For this review, take the finished solid that the model builds, in its own axes (mm). A direction names the side the tool comes from. Coordinates: 2 decimals unless noted, no trailing zeros. Order: outer loops, then holes, each group sorted by start corner. A loop starts at its lowest first (then second) coordinate and runs counter-clockwise, first axis right, second up. Notation, with made-up numbers: M 31.25,-31 L 42.25,-31 A34 cw 42.25,5 Z; hole C -1.5,17 d7. An arc over 180 degrees is marked long. Use CSV: the item, a comma, the result in double quotes.
```python
from build123d import *

# Parameters (mm, degrees)
EXTRUDE_1_DEPTH          = 5
SKETCH_2_W               = 67
SKETCH_2_H               = 34
EXTRUDE_2_DEPTH          = 5
SKETCH_4_W               = 57
SKETCH_4_H               = 57
EXTRUDE_3_DEPTH          = 5
CUT_EXTRUDE_1_DEPTH      = 5
FILLET_1_R               = 10
FILLET_2_R               = 10
SKETCH_6_R               = 1.25
SKETCH_6_R_2             = 12.5
CUT_EXTRUDE_2_DEPTH      = 5
PATTERN_CIRCULAR_1_COUNT = 4
SKETCH_7_R               = 1.25
CUT_EXTRUDE_3_DEPTH      = 5
SKETCH_8_R               = 1.25
CUT_EXTRUDE_5_DEPTH      = 10
PATTERN_CIRCULAR_2_COUNT = 3
PATTERN_CIRCULAR_2_ANGLE = 180


with BuildPart() as part:
    # 草图1 → 凸台-拉伸1 (new body)
    with BuildSketch(Plane.XY):
        Polygon((23, 17), (28, 17), (28, -17), (23, -17), (-5, -17), (-5, 17), align=None)
    extrude(amount=EXTRUDE_1_DEPTH)

    # 草图2 → 凸台-拉伸2 (add)
    with BuildSketch(Plane(origin=(28, 0, 0), x_dir=(0, 0, -1), z_dir=(1, 0, 0))):
        with Locations((-38.5, 0)):
            Rectangle(SKETCH_2_W, SKETCH_2_H)
    extrude(amount=-EXTRUDE_2_DEPTH)

    # 草图4 → 凸台-拉伸3 (add)
    with BuildSketch(Plane.ZY.offset(-23)):
        with Locations((43.5, 0)):
            Rectangle(SKETCH_4_W, SKETCH_4_H)
    extrude(amount=-EXTRUDE_3_DEPTH)

    # 草图5 → 切除-拉伸1 (cut)
    with BuildSketch(Plane.ZY.offset(-23)):
        with BuildLine():
            Line((15, 28.5), (15, 17))
            Line((15, 17), (20.625341533, 17))
            ThreePointArc((20.625341533, 17), (30.698632886, 25.463208753), (43.5, 28.5))
            Line((43.5, 28.5), (15, 28.5))
        make_face()
        with BuildLine():
            ThreePointArc((43.500000073, -28.5), (30.698632918, -25.463208769), (20.625341533, -17))
            Line((20.625341533, -17), (15, -17))
            Line((15, -17), (15, -28.5))
            Line((15, -28.5), (43.500000073, -28.5))
        make_face()
        with BuildLine():
            ThreePointArc((72, 0), (63.65254329, -20.152543238), (43.500000073, -28.5))
            Line((43.500000073, -28.5), (72, -28.5))
            Line((72, -28.5), (72, 0))
        make_face()
        with BuildLine():
            Line((72, 28.5), (43.5, 28.5))
            ThreePointArc((43.5, 28.5), (63.652543264, 20.152543264), (72, 0))
            Line((72, 0), (72, 28.5))
        make_face()
    extrude(amount=-CUT_EXTRUDE_1_DEPTH, mode=Mode.SUBTRACT)

    # 圆角1
    fillet_1_edges = [part.edges().sort_by_distance(p)[0] for p in [
        (25.5, 17, 20.625341533),
    ]]
    fillet(fillet_1_edges, radius=FILLET_1_R)

    # 圆角2
    fillet_2_edges = [part.edges().sort_by_distance(p)[0] for p in [
        (25.5, -17, 20.625341533),
    ]]
    fillet(fillet_2_edges, radius=FILLET_2_R)

    # 草图6 → 切除-拉伸2 (cut)
    with BuildSketch(Plane.ZY.offset(-23)):
        with Locations(Location((56.935028843, 13.435028843, 0), (0, 0, 270))):
            Circle(SKETCH_6_R)
        with Locations(Location((43.5, 0, 0), (0, 0, 270))):
            Circle(SKETCH_6_R_2)
    cut_extrude_2 = extrude(amount=-CUT_EXTRUDE_2_DEPTH, mode=Mode.SUBTRACT)

    # 阵列(圆周)1: 切除-拉伸2 ×4 about axis
    pattern_circular_1_axis = Axis((0, 0, 43.5), (1, 0, 0))
    for i in range(1, PATTERN_CIRCULAR_1_COUNT):
        add(cut_extrude_2.rotate(pattern_circular_1_axis, i * 360 / PATTERN_CIRCULAR_1_COUNT), mode=Mode.SUBTRACT)

    # 草图7 → 切除-拉伸3 (cut)
    with BuildSketch(Plane.XY.offset(5)):
        Circle(SKETCH_7_R)
        with Locations((0, 12)):
            Circle(SKETCH_7_R)
        with Locations(Location((0, -12, 0), (0, 0, 180))):
            Circle(SKETCH_7_R)
    extrude(amount=-CUT_EXTRUDE_3_DEPTH, mode=Mode.SUBTRACT)

    # 草图8 → 切除-拉伸5 (cut)
    with BuildSketch(Plane(origin=(28, 0, 0), x_dir=(0, 0, -1), z_dir=(1, 0, 0))):
        with Locations(Location((-43.5, 22.5, 0), (0, 0, 90))):
            Circle(SKETCH_8_R)
    cut_extrude_5 = extrude(amount=-CUT_EXTRUDE_5_DEPTH, mode=Mode.SUBTRACT)

    # 阵列(圆周)2: 切除-拉伸5 ×3 about axis
    pattern_circular_2_axis = Axis((0, 0, 43.5), (1, 0, 0))
    for i in range(1, PATTERN_CIRCULAR_2_COUNT):
        add(cut_extrude_5.rotate(pattern_circular_2_axis, i * PATTERN_CIRCULAR_2_ANGLE / (PATTERN_CIRCULAR_2_COUNT - 1)), mode=Mode.SUBTRACT)


solid = part.part
```
Item 1: To check wall thickness, follow line 1 along Y through (x, z) = (0, 3.5); line 2 along Z through (x, y) = (7, 12); line 3 along X through (y, z) = (11, 16). State the ranges of each line that lie inside material, in increasing order. Write a range as [from, to].
Solutions:
line 1,"[-17, -13.25], [-10.75, -1.25], [1.25, 10.75], [13.25, 17]"
line 2,"[0, 5]"
line 3,"[23, 28]"
Item 2: Draft analysis for pull direction X (two halves, no side actions). For faces 1 (the face through (-0.16, 13.24, 2.54)), 2 (the face through (25.535, 17.756, 19.868)), 3 (the face through (-5, 0, 2)), state which applies: released by +X, released by -X, zero draft, split by the parting line, or undercut.
Solutions:
face 1,"undercut"
face 2,"zero draft"
face 3,"released by -X"
Item 3: Add section D-D on y = -22.5. State the section outline as (x, z) points, and give its area (3 significant figures).
Solutions:
outline,"M 23,26.01 L 28,26.01 L 28,42.25 L 23,42.25 Z; M 23,44.75 L 28,44.75 L 28,60.99 L 23,60.99 Z"
area,"162 mm^2"
Item 4: Add section C-C on x = 25.5. State how many separate pieces and enclosed holes the cut face has, and give its area (3 significant figures).
Solutions:
separate pieces,"1"
enclosed holes,"8"
area,"2,600 mm^2"
Item 5: Clearance check with flat-ended pins moving along their axes: pin 1 Ø2 at (y, z) = (13.44, 56.94) entering from -X; pin 2 Ø8 at (x, y) = (18, 15.5) entering from +Z; pin 3 Ø4 at (x, z) = (23, 63) entering from -Y; pin 4 Ø4 at (x, y) = (24.5, -17) entering from +Z. State where each tip first meets the part, or that it passes through.
Solutions:
pin 1,"through"
pin 2,"z = 5"
pin 3,"y = -22.49"
pin 4,"z = 67.73"
Item 6: Add section B-B on z = 50. State the section outline as (x, y) points.
Solutions:
outline,"M 23,-27.75 L 28,-27.75 L 28,-10.68 L 23,-10.68 Z; M 23,10.68 L 28,10.68 L 28,27.75 L 23,27.75 Z"
Item 7: For faces 4 (the face through (12, 0, 0)), 5 (the face through (23, 0.4, 30.6)), 6 (the face through (15.4, -17, 4.6)), 7 (the face through (15.4, 17, 4.6)), list the 3-axis set-ups (+Z, -Z, +X, -X, +Y, -Y) from which the entire face can be reached by the end or side of a thin tool; tool diameter is ignored.
Solutions:
face 4,"-Z, +X, -X, +Y, -Y"
face 5,"+Z, -X, +Y, -Y"
face 6,"-Z, +X, -X, -Y"
face 7,"-Z, +X, -X, +Y"
Item 8: Add section A-A on x = 0. State the section outline as (y, z) points, and give its area (4 significant figures).
Solutions:
outline,"M -17,0 L -13.25,0 L -13.25,5 L -17,5 Z; M -10.75,0 L -1.25,0 L -1.25,5 L -10.75,5 Z; M 1.25,0 L 10.75,0 L 10.75,5 L 1.25,5 Z; M 13.25,0 L 17,0 L 17,5 L 13.25,5 Z"
area,"132.5 mm^2"
